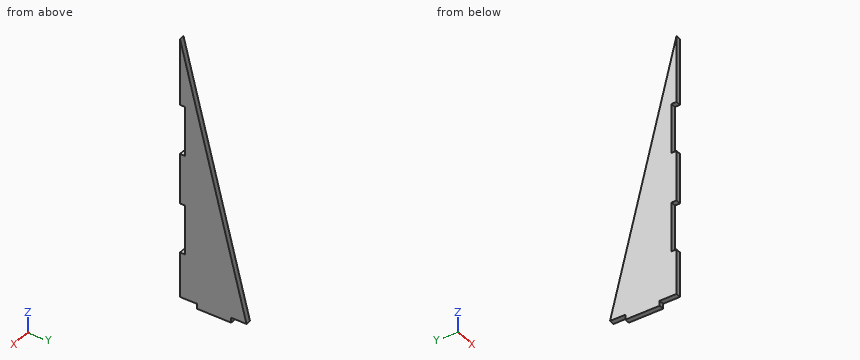
from build123d import *

# Parameters (mm, degrees)
BOSS_EXTRUDE1_DEPTH = 3


with BuildPart() as part:
    # Sketch2 → Boss-Extrude1 (new body)
    with BuildSketch(Plane(origin=(0, 0, 0), x_dir=(0, 0, -1), z_dir=(1, 0, 0))):
        Polygon((157, 39.25), (0, 0), (40.1, 0), (40.1, 3), (69.9, 3), (69.9, 0), (100.1, 0), (100.1, 3), (129.9, 3), (129.9, 0), (157, 0), (157, 10), (160, 10), (160, 30.2), (157, 30.2), align=None)
    extrude(amount=BOSS_EXTRUDE1_DEPTH)


solid = part.part
Read the model definition and answer for the solid it produces. Units are mm, in the model's axes. Round coordinates to 2 decimals unless told otherwise and drop trailing zeros. Write each loop counter-clockwise with the first axis right and the second up, starting at its lowest first coordinate (ties: lowest second). Pieces come first, ordered by that corner, then holes.
1. The part is cut by section A-A, the plane x = 2.2. Determine the outline of the cut face in (y, z), then the cut area to 3 significant figures.
2. The part is cut by section C-C, the plane y = 13. Determine the outline of the cut face in (x, z).
3. The part is cut by section B-B, the plane z = -80. Determine the outline of the cut face in (x, y).
4. Given pin 1 Ø1.5 at (x, y) = (1.5, 36.5) entering from -Z; pin 2 Ø0.9 at (x, z) = (1.5, -119.5) entering from -Y, each flat-ended and moving along its own axis, determine where each tip first touches the part or whether it passes through.
5. Straight lines are drawn through the part: L1, parallel to Y at x = 1.1, z = -40; L2, parallel to Y at x = 2, z = -15. For each, find the intervals that lie inside material, in ascending order.
Values:
1. outline: (0, -157) - (10, -157) - (10, -160) - (30.2, -160) - (30.2, -157) - (39.25, -157) - (0, 0) - (0, -40.1) - (3, -40.1) - (3, -69.9) - (0, -69.9) - (0, -100.1) - (3, -100.1) - (3, -129.9) - (0, -129.9) - close
1. area: 2,960 mm2
2. outline: (0, -160) - (3, -160) - (3, -52) - (0, -52) - close
3. outline: (0, 0) - (3, 0) - (3, 20) - (0, 20) - close
4. pin 1: stops at z = -157
4. pin 2: stops at y = 3
5. L1: y = 0 to 10
5. L2: y = 0 to 3.75
